from build123d import *

# Parameters (mm, degrees)
ESQUISSE1_W        = 250
ESQUISSE1_H        = 130
BOSS_EXTRU_1_DEPTH = 3.175
ESQUISSE2_W        = 3.175
ESQUISSE2_H        = 20
ESQUISSE2_W_2      = 20
ESQUISSE2_H_2      = 9.525
BOSS_EXTRU_2_DEPTH = 3.175


with BuildPart() as part:
    # Esquisse1 → Boss.-Extru.1 (new body)
    with BuildSketch(Plane(origin=(0, 0, 0), x_dir=(1, 0, 0), z_dir=(0, 1, 0))):
        with Locations((125, 65)):
            Rectangle(ESQUISSE1_W, ESQUISSE1_H)
    extrude(amount=BOSS_EXTRU_1_DEPTH)

    # Esquisse2 → Boss.-Extru.2 (add)
    with BuildSketch(Plane(origin=(0, 3.175, 0), x_dir=(1, 0, 0), z_dir=(0, 1, 0))):
        with Locations((-1.5875, 65)):
            Rectangle(ESQUISSE2_W, ESQUISSE2_H)
        with Locations((251.5875, 65)):
            Rectangle(ESQUISSE2_W, ESQUISSE2_H)
        with Locations((80, 134.7625)):
            Rectangle(ESQUISSE2_W_2, ESQUISSE2_H_2)
        with Locations((170, 134.7625)):
            Rectangle(ESQUISSE2_W_2, ESQUISSE2_H_2)
        with Locations((170, -4.7625)):
            Rectangle(ESQUISSE2_W_2, ESQUISSE2_H_2)
        with Locations((80, -4.7625)):
            Rectangle(ESQUISSE2_W_2, ESQUISSE2_H_2)
    extrude(amount=-BOSS_EXTRU_2_DEPTH)


solid = part.part
The listing builds one solid part. Answer for the finished solid, in the listing's coordinates (mm). Give positions to 0.01 mm unless a question says otherwise; leave off trailing zeros. Write each loop counter-clockwise with the first axis right and the second up, starting at its lowest first coordinate (ties: lowest second). Pieces come first, ordered by that corner, then holes. Notation, with made-up numbers: (16, 24) - (75, 24) arc R11 ccw to (75, 45) - close; hole circle Ø9 at (76.25, 73.5). An arc over 180 degrees is marked (long way). Use a Markdown table: item, result.
1. Section B-B on z = -116.5 is taken. Write down the section's boundary in (x, y) (3 decimals), plus the area to 3 significant figures.
Values follow:
| item | result |
|---|---|
| outline | (0, 0) - (250, 0) - (250, 3.175) - (0, 3.175) - close |
| area | 794 mm² |
2. Section C-C on x = 189 is taken. Write down the section's boundary in (y, z) (3 decimals), plus the area to 3 significant figures.
Values follow:
| item | result |
|---|---|
| outline | (0, -130) - (3.175, -130) - (3.175, 0) - (0, 0) - close |
| area | 413 mm² |
3. Each of these flat-tipped pins is pushed along its axis until it touches: P1, Ø1, axis at y = 1, z = 3.5, coming from the -X side; P2, Ø1, axis at x = 111, y = 2, coming from the -Z side; P3, Ø1.6, axis at x = 141.5, y = 1.5, coming from the +Z side. Where does it stop, or does it pass through?
Values follow:
| item | result |
|---|---|
| P1 | stops at x = 70 |
| P2 | stops at z = -130 |
| P3 | stops at z = 0 |
4. Find the intervals of material crossed by probe 1 along Z at (x, y) = (13, 0.5); probe 2 along X at (y, z) = (1.25, -93.5), in increasing order. Write a range as from..to.
Values follow:
| item | result |
|---|---|
| probe 1 | z = -130..0 |
| probe 2 | x = 0..250 |
5. Section A-A on y = 2.55 is taken. Write down the section's boundary in (x, z) (3 decimals).
Values follow:
| item | result |
|---|---|
| outline | (-3.175, -75) - (0, -75) - (0, -130) - (70, -130) - (70, -139.525) - (90, -139.525) - (90, -130) - (160, -130) - (160, -139.525) - (180, -139.525) - (180, -130) - (250, -130) - (250, -75) - (253.175, -75) - (253.175, -55) - (250, -55) - (250, 0) - (180, 0) - (180, 9.525) - (160, 9.525) - (160, 0) - (90, 0) - (90, 9.525) - (70, 9.525) - (70, 0) - (0, 0) - (0, -55) - (-3.175, -55) - close |
